from build123d import *

# Parameters (mm, degrees)
F0_W     = 500
F0_H     = 300
F1_DEPTH = 25
F2_W     = 50
F2_H     = 50
F3_DEPTH = 400
F4_W     = 50
F4_H     = 50
F5_DEPTH = 400
F7_DEPTH = 250


with BuildPart() as f1:
    # F0 (on Top) → F1 (new body)
    with BuildSketch(Plane.XY):
        with Locations((-45.115738, -73.622181)):
            Rectangle(F0_W, F0_H)
    extrude(amount=F1_DEPTH)

    # F2 (on face) → F3 (join)
    with BuildSketch(Plane(origin=(0, 0, 0), x_dir=(1, 0, 0), z_dir=(0, 0, -1))):
        with Locations((179.884262, -51.377819)):
            Rectangle(F2_W, F2_H)
        with Locations((179.884262, 198.622181)):
            Rectangle(F2_W, F2_H)
        with Locations((-270.115738, -51.377819)):
            Rectangle(F2_W, F2_H)
        with Locations((-270.115738, 198.622181)):
            Rectangle(F2_W, F2_H)
    extrude(amount=F3_DEPTH)

    # F4 (on face) → F5 (join)
    with BuildSketch(Plane.XY.offset(25)):
        with Locations((179.884262, -198.622181)):
            Rectangle(F4_W, F4_H)
        with Locations((-270.115738, -198.622181)):
            Rectangle(F4_W, F4_H)
    extrude(amount=F5_DEPTH)

    # F6 (on face) → F7 (join)
    with BuildSketch(Plane.XY.offset(425)):
        with BuildLine():
            Line((-245.115738, -173.622181), (-245.115738, -223.622181))
            ThreePointArc((-245.115738, -223.622181), (-44.389514, -258.960982), (156.33671, -223.622181))
            Line((156.33671, -223.622181), (155.415639, -173.622181))
            ThreePointArc((155.415639, -173.622181), (-44.850049, -195.2512), (-245.115738, -173.622181))
        make_face()
    extrude(amount=-F7_DEPTH)


solid = f1.part
Read the model definition and answer for the solid it produces. Units are mm, in the model's axes. A direction names the side the tool comes from. Round coordinates to 2 decimals unless told otherwise and drop trailing zeros. Write each loop counter-clockwise with the first axis right and the second up, starting at its lowest first coordinate (ties: lowest second). Pieces come first, ordered by that corner, then holes. Notation, with made-up numbers: M 58.25,-14.75 L 65.25,-14.75 A24 cw 65.25,6.25 Z; hole C 62.5,53.25 d4. An arc over 180 degrees is marked long. Use a Markdown table: item, result.
1) For a pull along Y with two mould halves and no side action, classify faces 1 (the flat face through (-270, -173.622, -197)), 2 (the flat face through (-28, -223.622, 11)), 3 (the cylindrical face through (-42.3, -195.248, 301.75)), 4 (the flat face through (-47, -216, 175)) as pulls with the +Y half, pulls with the -Y half, needs draft (parallel to the pull), parting line crosses it, or undercut.
Answers follow:
| item | result |
|---|---|
| face 1 | undercut |
| face 2 | pulls with the -Y half |
| face 3 | pulls with the +Y half |
| face 4 | needs draft |
2) Straight lines are drawn through the part: line 1 along Z through (x, y) = (-129.5, -199); line 2 along Z through (x, y) = (-14.5, -79); line 3 along Y through (x, z) = (-246, -143). For each, find the intervals that lie inside material, in ascending order. Write a range as [from, to].
Answers follow:
| item | result |
|---|---|
| line 1 | z = [0, 25], [175, 425] |
| line 2 | z = [0, 25] |
| line 3 | y = [-223.62, -173.62], [26.38, 76.38] |
3) The part is cut by section C-C (x = -105). Write down the section's boundary in (y, z).
Answers follow:
| item | result |
|---|---|
| outline | M -255.83,175 L -193.32,175 L -193.32,425 L -255.83,425 Z; M -223.62,0 L 76.38,0 L 76.38,25 L -223.62,25 Z |
4) The part is cut by section D-D (y = -184). Write down the section's boundary in (x, z).
Answers follow:
| item | result |
|---|---|
| outline | M -295.12,-400 L -245.12,-400 L -245.12,0 L 154.88,0 L 154.88,-400 L 204.88,-400 L 204.88,425 L 99.99,425 L 99.99,175 L 154.88,175 L 154.88,25 L -245.12,25 L -245.12,175 L -189.69,175 L -189.69,425 L -295.12,425 Z |
5) The part is cut by section A-A (z = 132.5). Write down the section's boundary in (x, y), plus the area to 3 significant figures.
Answers follow:
| item | result |
|---|---|
| outline | M -295.12,-223.62 L -245.12,-223.62 L -245.12,-173.62 L -295.12,-173.62 Z; M 154.88,-223.62 L 204.88,-223.62 L 204.88,-173.62 L 154.88,-173.62 Z |
| area | 5,000 mm2 |
6) A tool of negligible diameter and unlimited length cuts with its end or side. For faces 5 (the flat face through (-270, -173.622, 222)), 6 (the flat face through (180, -173.622, -197)), 7 (the flat face through (-49, -216, 425)), 8 (the flat face through (-245.116, -198, -197)), from which of +Z, -Z, +X, -X, +Y, -Y can it reach the whole face along a straight path? Write none if from no direction.
Answers follow:
| item | result |
|---|---|
| face 5 | +Z, +X, -X, +Y |
| face 6 | -Z, +X, -X |
| face 7 | +Z, +X, -X, +Y, -Y |
| face 8 | -Z, +Y, -Y |
7) The part is cut by section B-B (z = -282). Write down the section's boundary in (x, y).
Answers follow:
| item | result |
|---|---|
| outline | M -295.12,-223.62 L -245.12,-223.62 L -245.12,-173.62 L -295.12,-173.62 Z; M -295.12,26.38 L -245.12,26.38 L -245.12,76.38 L -295.12,76.38 Z; M 154.88,-223.62 L 204.88,-223.62 L 204.88,-173.62 L 154.88,-173.62 Z; M 154.88,26.38 L 204.88,26.38 L 204.88,76.38 L 154.88,76.38 Z |
8) Flat-ended cylindrical pins translate along their axes: pin 1 (15 mm diameter, centred on x = 190.5, z = -130, fed in from -Y); pin 2 (2 mm diameter, centred on x = -10.5, y = -62, fed in from +Z); pin 3 (25 mm diameter, centred on x = -262.5, z = 162, fed in from +Y). Find the tip coordinate at first contact, or state that the pin passes through.
Answers follow:
| item | result |
|---|---|
| pin 1 | stops at y = -223.62 |
| pin 2 | stops at z = 25 |
| pin 3 | stops at y = -173.62 |
